from build123d import *

# Parameters (mm, degrees)
SKETCH2_W           = 187.96
SKETCH2_H           = 152.4
BOSS_EXTRUDE1_DEPTH = 2.9718
SKETCH4_W           = 20.32
SKETCH4_H           = 3.048
SKETCH4_R           = 1.397
CUT_EXTRUDE1_DEPTH  = 5.08
BOSS_EXTRUDE2_DEPTH = 2.9718
FILLET1_R           = 5.08
CUT_EXTRUDE2_DEPTH  = 5.08
FILLET2_R           = 2.54
FILLET3_R           = 2.54
SKETCH7_R           = 1.397
CUT_EXTRUDE3_DEPTH  = 5.08
FILLET5_R           = 2.54
FILLET6_R           = 2.54


with BuildPart() as part:
    # Sketch2 → Boss-Extrude1 (new body)
    with BuildSketch(Plane(origin=(0, 0, 0), x_dir=(1, 0, 0), z_dir=(0, 1, 0))):
        with Locations((24.975168434, 0)):
            Rectangle(SKETCH2_W, SKETCH2_H)
    extrude(amount=BOSS_EXTRUDE1_DEPTH)

    # Sketch4 → Cut-Extrude1 (cut)
    with BuildSketch(Plane(origin=(0, 2.9718, 0), x_dir=(1, 0, 0), z_dir=(0, 1, 0))):
        with Locations((-46.144831566, -74.676)):
            Rectangle(SKETCH4_W, SKETCH4_H)
        with Locations((-46.144831566, 74.676)):
            Rectangle(SKETCH4_W, SKETCH4_H)
        with Locations((-13.124831566, -74.676)):
            Rectangle(SKETCH4_W, SKETCH4_H)
        with Locations((-13.124831566, 74.676)):
            Rectangle(SKETCH4_W, SKETCH4_H)
        with Locations((19.895168434, -74.676)):
            Rectangle(SKETCH4_W, SKETCH4_H)
        with Locations((19.895168434, 74.676)):
            Rectangle(SKETCH4_W, SKETCH4_H)
        with Locations((52.915168434, -74.676)):
            Rectangle(SKETCH4_W, SKETCH4_H)
        with Locations((52.915168434, 74.676)):
            Rectangle(SKETCH4_W, SKETCH4_H)
        with Locations(Location((82.125168434, -58.42, 0), (0, 0, 270))):
            Circle(SKETCH4_R)
        with Locations(Location((-10.330831566, -58.42, 0), (0, 0, 270))):
            Circle(SKETCH4_R)
        with Locations(Location((36.405168434, 74.422, 0), (0, 0, 270))):
            Circle(SKETCH4_R)
        with Locations(Location((3.385168434, 74.422, 0), (0, 0, 270))):
            Circle(SKETCH4_R)
        with Locations(Location((-29.634831566, 74.422, 0), (0, 0, 270))):
            Circle(SKETCH4_R)
        with Locations(Location((36.405168434, -74.422, 0), (0, 0, 270))):
            Circle(SKETCH4_R)
        with Locations(Location((3.385168434, -74.422, 0), (0, 0, 270))):
            Circle(SKETCH4_R)
        with Locations(Location((-29.634831566, -74.422, 0), (0, 0, 270))):
            Circle(SKETCH4_R)
        with Locations(Location((111.081256794, 69.85, 0), (0, 0, 270))):
            Circle(SKETCH4_R)
        with Locations(Location((111.081256794, -69.85, 0), (0, 0, 270))):
            Circle(SKETCH4_R)
        with Locations(Location((71.965256794, 69.85, 0), (0, 0, 270))):
            Circle(SKETCH4_R)
        with Locations(Location((71.965256794, -69.85, 0), (0, 0, 270))):
            Circle(SKETCH4_R)
        with Locations(Location((82.125168434, 34.036, 0), (0, 0, 270))):
            Circle(SKETCH4_R)
        with Locations(Location((-10.330831566, 34.036, 0), (0, 0, 270))):
            Circle(SKETCH4_R)
    extrude(amount=-CUT_EXTRUDE1_DEPTH, mode=Mode.SUBTRACT)

    # Sketch5 → Boss-Extrude2 (add)
    with BuildSketch(Plane(origin=(0, 2.9718, 0), x_dir=(1, 0, 0), z_dir=(0, 1, 0))):
        with BuildLine():
            ThreePointArc((38.185030781, 76.2), (36.405168434, 76.937788936), (34.625306088, 76.2))
            Line((34.625306088, 76.2), (38.185030781, 76.2))
        make_face()
        with BuildLine():
            Line((1.605306088, 76.2), (5.165030781, 76.2))
            ThreePointArc((5.165030781, 76.2), (3.385168434, 76.937788936), (1.605306088, 76.2))
        make_face()
        with BuildLine():
            Line((-31.414693912, 76.2), (-27.854969219, 76.2))
            ThreePointArc((-27.854969219, 76.2), (-29.634831566, 76.937788936), (-31.414693912, 76.2))
        make_face()
        with BuildLine():
            ThreePointArc((-31.414693912, -76.2), (-29.634831566, -76.937788936), (-27.854969219, -76.2))
            Line((-27.854969219, -76.2), (-31.414693912, -76.2))
        make_face()
        with BuildLine():
            ThreePointArc((1.605306088, -76.2), (3.385168434, -76.937788936), (5.165030781, -76.2))
            Line((5.165030781, -76.2), (1.605306088, -76.2))
        make_face()
        with BuildLine():
            ThreePointArc((34.625306088, -76.2), (36.405168434, -76.937788936), (38.185030781, -76.2))
            Line((38.185030781, -76.2), (34.625306088, -76.2))
        make_face()
    extrude(amount=-BOSS_EXTRUDE2_DEPTH)

    # Fillet1
    fillet1_edges = [part.edges().sort_by_distance(p)[0] for p in [
        (118.955168434, 1.4859, 76.2),
        (118.955168434, 1.4859, -76.2),
    ]]
    fillet(fillet1_edges, radius=FILLET1_R)

    # Sketch6 → Cut-Extrude2 (cut)
    with BuildSketch(Plane(origin=(0, 2.9718, 0), x_dir=(1, 0, 0), z_dir=(0, 1, 0))):
        Polygon((118.955168434, -98.380031514), (118.955168434, -65.024), (101.175168434, -65.024), (101.175168434, -51.308), (89.237168434, -51.308), (89.237168434, 51.308), (101.175168434, 51.308), (101.175168434, 65.024), (118.955168434, 65.024), (118.955168434, 98.380031514), (174.761445674, 98.380031514), (174.761445674, -98.380031514), align=None)
    extrude(amount=-CUT_EXTRUDE2_DEPTH, mode=Mode.SUBTRACT)

    # Fillet2
    fillet2_edges = [part.edges().sort_by_distance(p)[0] for p in [
        (101.175168434, 1.4859, -51.308),
    ]]
    fillet(fillet2_edges, radius=FILLET2_R)

    # Fillet3
    fillet3_edges = [part.edges().sort_by_distance(p)[0] for p in [
        (101.175168434, 1.4859, 65.024),
        (101.175168434, 1.4859, 51.308),
        (118.955168434, 1.4859, 65.024),
        (101.175168434, 1.4859, -65.024),
        (118.955168434, 1.4859, -65.024),
    ]]
    fillet(fillet3_edges, radius=FILLET3_R)

    # Sketch7 → Cut-Extrude3 (cut)
    with BuildSketch(Plane(origin=(0, 2.9718, 0), x_dir=(1, 0, 0), z_dir=(0, 1, 0))):
        with Locations(Location((-51.986831566, 19.304, 0), (0, 0, 270))):
            Circle(SKETCH7_R)
        with Locations(Location((-51.986831566, -19.304, 0), (0, 0, 270))):
            Circle(SKETCH7_R)
    extrude(amount=-CUT_EXTRUDE3_DEPTH, mode=Mode.SUBTRACT)

    # Fillet5
    fillet5_edges = [part.edges().sort_by_distance(p)[0] for p in [
        (89.237168434, 1.4859, -51.308),
    ]]
    fillet(fillet5_edges, radius=FILLET5_R)

    # Fillet6
    fillet6_edges = [part.edges().sort_by_distance(p)[0] for p in [
        (89.237168434, 1.4859, 51.308),
    ]]
    fillet(fillet6_edges, radius=FILLET6_R)


solid = part.part
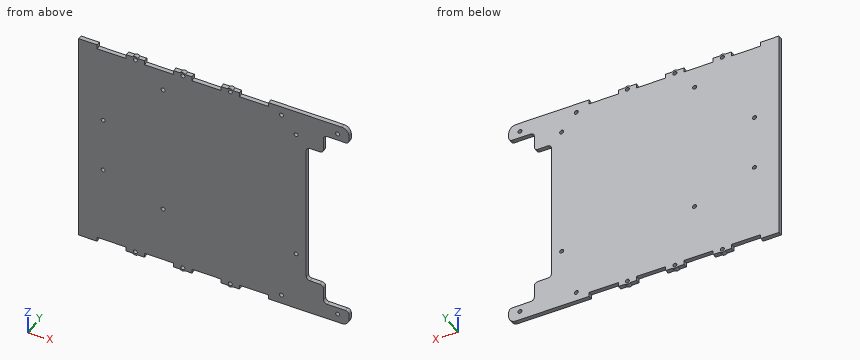
Geometry: final body of the model. Coordinates: model frame, mm. Coordinates: 2 decimals unless noted, no trailing zeros. One line per item, written item: value. Start each with the question number.
1) Cut plane A-A (y = 1.25). Count the separate pieces of the cut face and the enclosed holes in it, then the cut area to 3 significant figures.
2) Pin query (flat end, axial travel): P1, Ø0.9, axis at x = -1.5, y = 1, coming from the +Z side; P2, Ø1.7, axis at x = 3.39, z = 74.42, coming from the -Y side; P3, Ø0.9, axis at y = 1, z = -74, coming from the +X side; P4, Ø1.5, axis at y = 2, z = 74.5, coming from the +X side. Return the tip coordinate at first contact, or that it passes through.
3) Material intervals for L1, parallel to X at y = 1.5, z = 69.85; L2, parallel to Z at x = 97.5, y = 0.6; L3, parallel to Z at x = -52.5, y = 2.85, sorted ascending. Write a range as from..to.
Evaluation:
1. separate pieces: 1
1. enclosed holes: 16
1. area: 24,500 mm^2
2. P1: z = 76.2
2. P2: through
2. P3: x = 118.34
2. P4: x = 118.22
3. L1: -69..70.57, 73.36..109.68, 112.48..118.96
3. L2: -76.2..-51.31, 51.31..76.2
3. L3: -73.15..-20.6, -18..18, 20.6..73.15
